from build123d import *

# Parameters (mm, degrees)
SKETCH1_W                    = 120
SKETCH1_H                    = 265
BOSS_EXTRUDE1_DEPTH          = 42
CHAMFER1_SIZE                = 30
FILLET3_R                    = 25
SHELL1_T                     = -4
FILLET4_R                    = 5
BOSS_EXTRUDE2_DEPTH          = 15
BOSS_EXTRUDE2_DEPTH_BACK     = 42
FILLET7_R                    = 5
SKETCH4_W                    = 128
SKETCH4_H                    = 4
CUT_EXTRUDE1_DEPTH           = 236.172277278
CSK_FOR_M3_SFHCS1_AT_2_COUNT = 2
CSK_FOR_M3_SFHCS1_AT_2_PITCH = 50
CSK_FOR_M3_SFHCS1_AT_3_COUNT = 2
CSK_FOR_M3_SFHCS1_AT_3_PITCH = 100
CSK_FOR_M3_SFHCS1_AT_4_COUNT = 2
CSK_FOR_M3_SFHCS1_AT_4_PITCH = 150
CSK_FOR_M3_SFHCS1_AT_5_COUNT = 2
CSK_FOR_M3_SFHCS1_AT_5_PITCH = 200
SKETCH7_W                    = 112
SKETCH7_H                    = 20.766378669
CUT_EXTRUDE2_DEPTH           = 231.4994577


with BuildPart() as part:
    # Sketch1 → Boss-Extrude1 (new body)
    with BuildSketch(Plane.XY):
        with Locations((0, 82.5)):
            Rectangle(SKETCH1_W, SKETCH1_H)
    extrude(amount=BOSS_EXTRUDE1_DEPTH)

    # Chamfer1
    chamfer1_edges = [part.edges().sort_by_distance(p)[0] for p in [
        (60, -50, 21),
        (-60, -50, 21),
    ]]
    chamfer(chamfer1_edges, length=CHAMFER1_SIZE)

    # Fillet3
    fillet3_edges = [part.edges().sort_by_distance(p)[0] for p in [
        (30, -50, 21),
        (-30, -50, 21),
        (-60, -20, 21),
        (60, -20, 21),
    ]]
    fillet(fillet3_edges, radius=FILLET3_R)

    # Shell1
    shell1_openings = [part.faces().sort_by_distance(p)[0] for p in [
        (0, 86.277211475, 42),
    ]]
    offset(amount=SHELL1_T, openings=shell1_openings, kind=Kind.INTERSECTION)

    # Fillet4
    fillet4_edges = [part.edges().sort_by_distance(p)[0] for p in [
        (-56, 211, 23),
        (56, 211, 23),
    ]]
    fillet(fillet4_edges, radius=FILLET4_R)

    # Sketch2 → Boss-Extrude2 (add, two sides: drawn at the far end of the back side and taken through both)
    with BuildSketch(Plane.XY.offset(42).offset(-BOSS_EXTRUDE2_DEPTH_BACK)):
        with BuildLine():
            Line((-64, 219), (-64, -9.644660941))
            ThreePointArc((-64, -9.644660941), (-61.792506443, -20.742480479), (-55.506096654, -30.150757595))
            Line((-55.506096654, -30.150757595), (-40.150757595, -45.506096654))
            ThreePointArc((-40.150757595, -45.506096654), (-30.742480479, -51.792506443), (-19.644660941, -54))
            Line((-19.644660941, -54), (19.644660941, -54))
            ThreePointArc((19.644660941, -54), (30.742480479, -51.792506443), (40.150757595, -45.506096654))
            Line((40.150757595, -45.506096654), (55.506096654, -30.150757595))
            ThreePointArc((55.506096654, -30.150757595), (61.792506443, -20.742480479), (64, -9.644660941))
            Line((64, -9.644660941), (64, 219))
            Line((64, 219), (-64, 219))
        make_face()
        with BuildLine():
            Line((-60, 215), (-60, -9.644660941))
            ThreePointArc((-60, -9.644660941), (-58.096988313, -19.21174675), (-52.67766953, -27.32233047))
            Line((-52.67766953, -27.32233047), (-37.32233047, -42.67766953))
            ThreePointArc((-37.32233047, -42.67766953), (-29.21174675, -48.096988313), (-19.644660941, -50))
            Line((-19.644660941, -50), (19.644660941, -50))
            ThreePointArc((19.644660941, -50), (29.21174675, -48.096988313), (37.32233047, -42.67766953))
            Line((37.32233047, -42.67766953), (52.67766953, -27.32233047))
            ThreePointArc((52.67766953, -27.32233047), (58.096988313, -19.21174675), (60, -9.644660941))
            Line((60, -9.644660941), (60, 215))
            Line((60, 215), (-60, 215))
        make_face(mode=Mode.SUBTRACT)
    extrude(amount=BOSS_EXTRUDE2_DEPTH + BOSS_EXTRUDE2_DEPTH_BACK)

    # Fillet7
    fillet7_edges = [part.edges().sort_by_distance(p)[0] for p in [
        (0, 219, 0),
        (64, 104.67766953, 0),
        (61.792506443, -20.742480479, 0),
        (47.828427125, -37.828427125, 0),
        (30.742480479, -51.792506443, 0),
        (0, -54, 0),
        (-30.742480479, -51.792506443, 0),
        (-47.828427125, -37.828427125, 0),
        (-61.792506443, -20.742480479, 0),
        (-64, 104.67766953, 0),
    ]]
    fillet(fillet7_edges, radius=FILLET7_R)

    # Sketch4 → Cut-Extrude1 (cut, through all)
    with BuildSketch(Plane.XY.offset(57)):
        with Locations((0, 217)):
            Rectangle(SKETCH4_W, SKETCH4_H)
    extrude(amount=-CUT_EXTRUDE1_DEPTH, mode=Mode.SUBTRACT)

    # Sketch6 → CSK for M3 SFHCS1 (revolve, cut)
    with BuildSketch(Plane(origin=(-64, 7.5, 49.5), x_dir=(0, 0, 1), z_dir=(0, 1, 0))):
        Polygon((0, 0), (0, 16.021463052), (1.7, 15), (1.7, 1.66), (3.36, 0), align=None)
    csk_for_m3_sfhcs1 = revolve(axis=Axis((-70.35, 7.5, 49.5), (1, 0, 0)), mode=Mode.SUBTRACT)

    # CSK for M3 SFHCS1 at 2: CSK for M3 SFHCS1 ×2
    with Locations(*[(0, i * CSK_FOR_M3_SFHCS1_AT_2_PITCH, 0) for i in range(1, CSK_FOR_M3_SFHCS1_AT_2_COUNT)]):
        add(csk_for_m3_sfhcs1, mode=Mode.SUBTRACT)

    # CSK for M3 SFHCS1 at 3: CSK for M3 SFHCS1 ×2
    with Locations(*[(0, i * CSK_FOR_M3_SFHCS1_AT_3_PITCH, 0) for i in range(1, CSK_FOR_M3_SFHCS1_AT_3_COUNT)]):
        add(csk_for_m3_sfhcs1, mode=Mode.SUBTRACT)

    # CSK for M3 SFHCS1 at 4: CSK for M3 SFHCS1 ×2
    with Locations(*[(0, i * CSK_FOR_M3_SFHCS1_AT_4_PITCH, 0) for i in range(1, CSK_FOR_M3_SFHCS1_AT_4_COUNT)]):
        add(csk_for_m3_sfhcs1, mode=Mode.SUBTRACT)

    # CSK for M3 SFHCS1 at 5: CSK for M3 SFHCS1 ×2
    with Locations(*[(0, i * CSK_FOR_M3_SFHCS1_AT_5_PITCH, 0) for i in range(1, CSK_FOR_M3_SFHCS1_AT_5_COUNT)]):
        add(csk_for_m3_sfhcs1, mode=Mode.SUBTRACT)

    # Mirror1: CSK for M3 SFHCS1 across plane
    add(csk_for_m3_sfhcs1.mirror(Plane(origin=(0, 0, 0), x_dir=(0, 0, 1), z_dir=(1, 0, 0))), mode=Mode.SUBTRACT)

    # Mirror1 copy 1 sketch → Mirror1 copy 1 (revolve, cut)
    with BuildSketch(Plane(origin=(64, 57.5, 49.5), x_dir=(0, 0, 1), z_dir=(0, 1, 0))):
        Polygon((0, 0), (0, -16.021463052), (1.7, -15), (1.7, -1.66), (3.36, 0), align=None)
    revolve(axis=Axis((70.35, 57.5, 49.5), (1, 0, 0)), mode=Mode.SUBTRACT)

    # Mirror1 copy 2 sketch → Mirror1 copy 2 (revolve, cut)
    with BuildSketch(Plane(origin=(64, 107.5, 49.5), x_dir=(0, 0, 1), z_dir=(0, 1, 0))):
        Polygon((0, 0), (0, -16.021463052), (1.7, -15), (1.7, -1.66), (3.36, 0), align=None)
    revolve(axis=Axis((70.35, 107.5, 49.5), (1, 0, 0)), mode=Mode.SUBTRACT)

    # Mirror1 copy 3 sketch → Mirror1 copy 3 (revolve, cut)
    with BuildSketch(Plane(origin=(64, 157.5, 49.5), x_dir=(0, 0, 1), z_dir=(0, 1, 0))):
        Polygon((0, 0), (0, -16.021463052), (1.7, -15), (1.7, -1.66), (3.36, 0), align=None)
    revolve(axis=Axis((70.35, 157.5, 49.5), (1, 0, 0)), mode=Mode.SUBTRACT)

    # Mirror1 copy 4 sketch → Mirror1 copy 4 (revolve, cut)
    with BuildSketch(Plane(origin=(64, 207.5, 49.5), x_dir=(0, 0, 1), z_dir=(0, 1, 0))):
        Polygon((0, 0), (0, -16.021463052), (1.7, -15), (1.7, -1.66), (3.36, 0), align=None)
    revolve(axis=Axis((70.35, 207.5, 49.5), (1, 0, 0)), mode=Mode.SUBTRACT)

    # Sketch7 → Cut-Extrude2 (cut, through all)
    with BuildSketch(Plane.XY.offset(4)):
        with Locations((0, 202.616810665)):
            Rectangle(SKETCH7_W, SKETCH7_H)
    extrude(amount=CUT_EXTRUDE2_DEPTH, mode=Mode.SUBTRACT)


solid = part.part
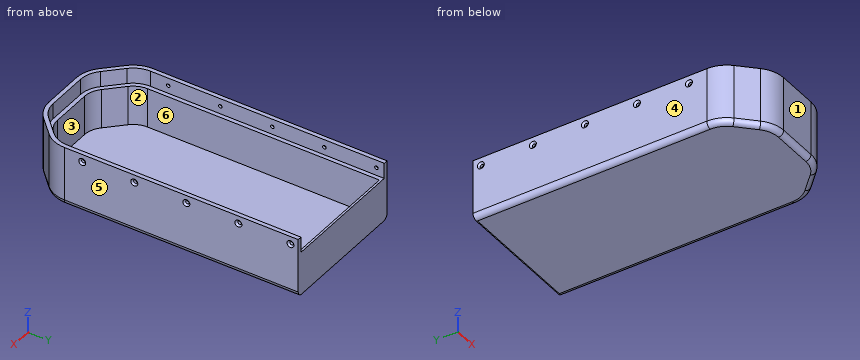
Geometry: final body of the model. Coordinates: model frame, mm. Face numbers are marked on the shaded views. A direction names the side the tool comes from. Coordinates: 2 decimals unless noted, no trailing zeros. Loops run counter-clockwise (first coordinate to the right, second up) from the corner with the lowest first, then second, coordinate; pieces in that order, holes last. Notation, with made-up numbers: (24, -31.75) - (47, -31.75) arc R15 cw to (47, -15.75) - close; hole circle Ø2 at (65, -23). An arc over 180 degrees is marked (long way). One line per question, with ' | ' between items. Start each with the question number.
(1) Cut plane B-B on x = -1. Output: boundary loops of the cut face in (y, z).
(2) Reachability of the marked faces 1 and 2 from +Z, -Z, +X, -X, +Y, -Y: full face, straight path, thin tool, end or side. Return the list, or none.
(3) First-contact query: pin 1 (7.5 mm diameter, centred on x = -7.5, z = 47.5, fed in from +Y); pin 2 (4 mm diameter, centred on x = -22, y = 167, fed in from +Z); pin 3 (10 mm diameter, centred on x = -37.5, z = 27.5, fed in from -Y) (3 decimals); pin 4 (2.5 mm diameter, centred on y = 207.5, z = 49.5, fed in from +X). Flat tips, straight axial feed; report the tip coordinate or a pass-through.
(4) Cut plane A-A on z = 24. Output: boundary loops of the cut face in (x, y), and give its area (3 significant figures).
(5) Draft query along X for the marked faces 3, 4, 5 and 6. Return one class per face: +X half, -X half, draft (parallel to the pull), parting line (faces both ways), or undercut.
(6) Cut plane C-C on y = 84. Output: boundary loops of the cut face in (x, z), and give its area (3 significant figures).
(7) Ray query, L1, parallel to X at y = 196, z = 54; L2, parallel to Y at x = -4.5, z = 33; L3, parallel to X at y = 179.5, z = 37. Return the intervals inside material, ascending. Write a range as from..to.
Here are the results:
1) outline: (-54, 5) arc R5 ccw to (-49, 0) - (214, 0) arc R5 ccw to (215, 0.1) - (215, 42) - (213, 42) - (213, 4) - (-46, 4) - (-46, 42) - (-50, 42) - (-50, 57) - (-54, 57) - close
2) face 1: +Z, -Z, +X, -X, -Y | face 2: +Z
3) pin 1: y = -50 | pin 2: z = 4 | pin 3: y = -50.995 | pin 4: through
4) outline: (-64, -9.64) arc R29 ccw to (-55.51, -30.15) - (-40.15, -45.51) arc R29 ccw to (-19.64, -54) - (19.64, -54) arc R29 ccw to (40.15, -45.51) - (55.51, -30.15) arc R29 ccw to (64, -9.64) - (64, 215) - (-64, 215) - close; hole (-56, -9.64) arc R21 ccw to (-49.85, -24.49) - (-34.49, -39.85) arc R21 ccw to (-19.64, -46) - (19.64, -46) arc R21 ccw to (34.49, -39.85) - (49.85, -24.49) arc R21 ccw to (56, -9.64) - (56, 213) - (-56, 213) - close | area: 5,110 mm²
5) face 3: undercut | face 4: -X half | face 5: +X half | face 6: undercut
6) outline: (-64, 5) arc R5 ccw to (-59, 0) - (59, 0) arc R5 ccw to (64, 5) - (64, 57) - (60, 57) - (60, 42) - (56, 42) - (56, 4) - (-56, 4) - (-56, 42) - (-60, 42) - (-60, 57) - (-64, 57) - close | area: 1,230 mm²
7) L1: -64..-60, 60..64 | L2: -54..-46, 213..215 | L3: -64..-56, 56..64
